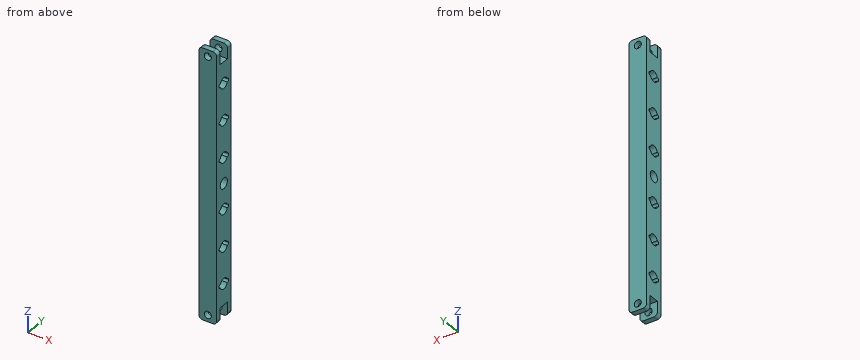
from build123d import *

# Parameters (mm, degrees)
SKETCH1_W           = 863.6
SKETCH1_H           = 76.2
BOSS_EXTRUDE1_DEPTH = 63.5
SKETCH2_R           = 19.05
CUT_EXTRUDE1_DEPTH  = 63.5
SKETCH3_W           = 63.5
SKETCH3_H           = 19.05
BOSS_EXTRUDE2_DEPTH = 50.8
SKETCH4_W           = 63.5
SKETCH4_H           = 19.05
BOSS_EXTRUDE3_DEPTH = 50.8
SKETCH5_R           = 12.7
CUT_EXTRUDE2_DEPTH  = 221.742
FILLET1_R           = 12.7


with BuildPart() as part:
    # Sketch1 → Boss-Extrude1 (new body)
    with BuildSketch(Plane(origin=(0, 0, 0), x_dir=(0, 0, -1), z_dir=(1, 0, 0))):
        Rectangle(SKETCH1_W, SKETCH1_H)
        with BuildLine():
            ThreePointArc((-362.147128046, 17.991666667), (-374.935943609, 0), (-362.147128046, -17.991666667))
            ThreePointArc((-362.147128046, -17.991666667), (-355.885943609, -25.4), (-349.624759172, -17.991666667))
            ThreePointArc((-349.624759172, -17.991666667), (-336.835943609, 0), (-349.624759172, 17.991666667))
            ThreePointArc((-349.624759172, 17.991666667), (-355.885943609, 25.4), (-362.147128046, 17.991666667))
        make_face(mode=Mode.SUBTRACT)
        with BuildLine():
            ThreePointArc((-230.067128046, 17.991666667), (-242.855943609, 0), (-230.067128046, -17.991666667))
            ThreePointArc((-230.067128046, -17.991666667), (-223.805943609, -25.4), (-217.544759172, -17.991666667))
            ThreePointArc((-217.544759172, -17.991666667), (-204.755943609, 0), (-217.544759172, 17.991666667))
            ThreePointArc((-217.544759172, 17.991666667), (-223.805943609, 25.4), (-230.067128046, 17.991666667))
        make_face(mode=Mode.SUBTRACT)
        with BuildLine():
            ThreePointArc((-96.728869239, 18.381328438), (-110.775943609, 0), (-96.728869239, -18.381328438))
            ThreePointArc((-96.728869239, -18.381328438), (-89.970708805, -25.339280787), (-84.23643534, -17.51598601))
            ThreePointArc((-84.23643534, -17.51598601), (-72.675943609, 0), (-84.23643534, 17.51598601))
            ThreePointArc((-84.23643534, 17.51598601), (-89.970708805, 25.339280787), (-96.728869239, 18.381328438))
        make_face(mode=Mode.SUBTRACT)
        with BuildLine():
            ThreePointArc((84.23643534, -17.51598601), (72.675943609, 0), (84.23643534, 17.51598601))
            ThreePointArc((84.23643534, 17.51598601), (89.970708805, 25.339280787), (96.728869239, 18.381328438))
            ThreePointArc((96.728869239, 18.381328438), (110.775943609, 0), (96.728869239, -18.381328438))
            ThreePointArc((96.728869239, -18.381328438), (89.970708805, -25.339280787), (84.23643534, -17.51598601))
        make_face(mode=Mode.SUBTRACT)
        with BuildLine():
            ThreePointArc((217.544759172, -17.991666667), (204.755943609, 0), (217.544759172, 17.991666667))
            ThreePointArc((217.544759172, 17.991666667), (223.805943609, 25.4), (230.067128046, 17.991666667))
            ThreePointArc((230.067128046, 17.991666667), (242.855943609, 0), (230.067128046, -17.991666667))
            ThreePointArc((230.067128046, -17.991666667), (223.805943609, -25.4), (217.544759172, -17.991666667))
        make_face(mode=Mode.SUBTRACT)
        with BuildLine():
            ThreePointArc((349.624759172, -17.991666667), (336.835943609, 0), (349.624759172, 17.991666667))
            ThreePointArc((349.624759172, 17.991666667), (355.885943609, 25.4), (362.147128046, 17.991666667))
            ThreePointArc((362.147128046, 17.991666667), (374.935943609, 0), (362.147128046, -17.991666667))
            ThreePointArc((362.147128046, -17.991666667), (355.885943609, -25.4), (349.624759172, -17.991666667))
        make_face(mode=Mode.SUBTRACT)
    extrude(amount=BOSS_EXTRUDE1_DEPTH)

    # Sketch2 → Cut-Extrude1 (cut)
    with BuildSketch(Plane(origin=(63.5, 0, 0), x_dir=(0, 0, -1), z_dir=(1, 0, 0))):
        Circle(SKETCH2_R)
    extrude(amount=-CUT_EXTRUDE1_DEPTH, mode=Mode.SUBTRACT)

    # Sketch3 → Boss-Extrude2 (add)
    with BuildSketch(Plane(origin=(0, 0, -431.8), x_dir=(-1, 0, 0), z_dir=(0, 0, -1))):
        with Locations((-31.75, 28.575)):
            Rectangle(SKETCH3_W, SKETCH3_H)
        with Locations((-31.75, -28.575)):
            Rectangle(SKETCH3_W, SKETCH3_H)
    extrude(amount=BOSS_EXTRUDE2_DEPTH)

    # Sketch4 → Boss-Extrude3 (add)
    with BuildSketch(Plane.XY.offset(431.8)):
        with Locations((31.75, -28.575)):
            Rectangle(SKETCH4_W, SKETCH4_H)
        with Locations((31.75, 28.575)):
            Rectangle(SKETCH4_W, SKETCH4_H)
    extrude(amount=BOSS_EXTRUDE3_DEPTH)

    # Sketch5 → Cut-Extrude2 (cut)
    with BuildSketch(Plane(origin=(0, 38.1, 0), x_dir=(1, 0, 0), z_dir=(0, 1, 0))):
        with Locations(Location((31.75, 458.42897264, 0), (0, 0, 270))):
            Circle(SKETCH5_R)
        with Locations(Location((31.75, -458.42897264, 0), (0, 0, 270))):
            Circle(SKETCH5_R)
    extrude(amount=-CUT_EXTRUDE2_DEPTH, mode=Mode.SUBTRACT)

    # Fillet1
    fillet1_edges = [part.edges().sort_by_distance(p)[0] for p in [
        (0, -28.575, -482.6),
        (63.5, -28.575, -482.6),
        (63.5, 28.575, -482.6),
        (0, 28.575, -482.6),
        (0, 28.575, 482.6),
        (63.5, 28.575, 482.6),
        (63.5, -28.575, 482.6),
        (0, -28.575, 482.6),
    ]]
    fillet(fillet1_edges, radius=FILLET1_R)


solid = part.part
CAD build for the part. Positions are in the model's coordinates, mm. Round coordinates to 2 decimals unless told otherwise and drop trailing zeros. Write each loop counter-clockwise with the first axis right and the second up, starting at its lowest first coordinate (ties: lowest second). Pieces come first, ordered by that corner, then holes. Notation, with made-up numbers: M -15,7.25 L 25,7.25 A24 ccw 25,31.25 Z; hole C -18,3 d4. An arc over 180 degrees is marked long. Put each result on its own line as item: value. Start each with the question number.
1) Pin check, flat tips, straight feed: pin 1 Ø8 at (x, y) = (17.5, 2.5) entering from +Z; pin 2 Ø1 at (x, y) = (39.5, -4.5) entering from -Z; pin 3 Ø11.5 at (y, z) = (-19, -90.41) entering from +X. Stop position of each tip, or through.
2) Saw through at A-A, the plane y = 0. Count the separate pieces of the cut face and the enclosed holes in it, and give its area (3 significant figures).
3) Drill centre lines: probe 1 along Z at (x, y) = (31, -31); probe 2 along Y at (x, z) = (31.5, 433); probe 3 along Y at (x, z) = (27, -348.5). Where is each one in solid material? Low to high. Write a range as [from, to].
4) Saw through at B-B, the plane z = 0. Write the cut outline in (x, y), and give its area (3 significant figures).
Resolved:
1. pin 1: z = 431.8
1. pin 2: z = -431.8
1. pin 3: through
2. separate pieces: 8
2. enclosed holes: 0
2. area: 37,900 mm²
3. probe 1: [-482.6, -471.11], [-445.75, 445.75], [471.11, 482.6]
3. probe 2: [-38.1, -19.05], [19.05, 38.1]
3. probe 3: [-38.1, -17.56], [17.56, 38.1]
4. outline: M 0,-38.1 L 63.5,-38.1 L 63.5,-19.05 L 0,-19.05 Z; M 0,19.05 L 63.5,19.05 L 63.5,38.1 L 0,38.1 Z
4. area: 2,420 mm²
